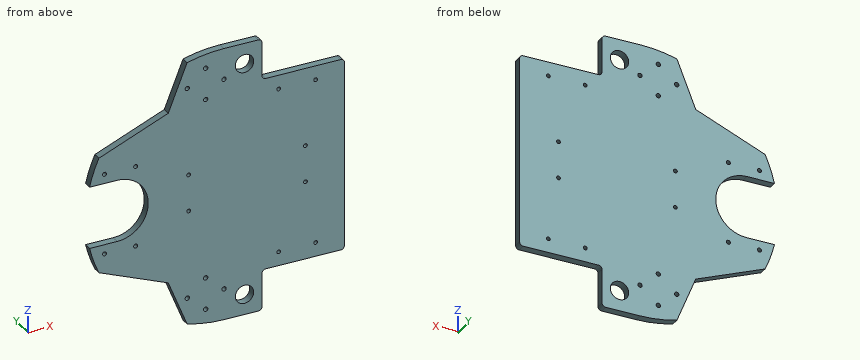
from build123d import *

# Parameters (mm, degrees)
BOSS_EXTRUDE1_DEPTH = 6.35
SKETCH8_R           = 1.651
CUT_EXTRUDE5_DEPTH  = 162.484606465
CUT_EXTRUDE6_DEPTH  = 160.416662013
SKETCH16_R          = 1.775
CUT_EXTRUDE9_DEPTH  = 160.416662013
SKETCH17_R          = 1.55
SKETCH17_R_2        = 7.5
SKETCH17_W          = 67.26995632
SKETCH17_H          = 33.5
CUT_EXTRUDE10_DEPTH = 160.416662013
FILLET1_R           = 3
SKETCH18_R          = 1.55
CUT_EXTRUDE11_DEPTH = 160.416662013


with BuildPart() as part:
    # Sketch1 → Boss-Extrude1 (new body)
    with BuildSketch(Plane(origin=(0, 0, 0), x_dir=(1, 0, 0), z_dir=(0, 1, 0))):
        with BuildLine():
            Line((-3.175, 112.5), (95.25, 112.5))
            Line((95.25, 112.5), (95.25, -112.5))
            Line((95.25, -112.5), (-3.175, -112.5))
            ThreePointArc((-3.175, -112.5), (-115.675, 0), (-3.175, 112.5))
        make_face()
    extrude(amount=-BOSS_EXTRUDE1_DEPTH)

    # Sketch8 → Cut-Extrude5 (cut, through all)
    with BuildSketch(Plane(origin=(0, 0, 0), x_dir=(1, 0, 0), z_dir=(0, 1, 0))):
        with Locations(Location((-100.5586, 33.02, 0), (0, 0, 270))):
            Circle(SKETCH8_R)
        with Locations(Location((-100.5586, -33.02, 0), (0, 0, 270))):
            Circle(SKETCH8_R)
        with Locations(Location((-75.1586, 33.02, 0), (0, 0, 270))):
            Circle(SKETCH8_R)
        with Locations(Location((-75.1586, -33.02, 0), (0, 0, 270))):
            Circle(SKETCH8_R)
        with BuildLine():
            Line((-90.2716, 25.4), (-229.776686608, 25.4))
            Line((-229.776686608, 25.4), (-229.776686608, -25.4))
            Line((-229.776686608, -25.4), (-90.2716, -25.4))
            ThreePointArc((-90.2716, -25.4), (-64.8716, 0), (-90.2716, 25.4))
        make_face()
    extrude(amount=-CUT_EXTRUDE5_DEPTH, mode=Mode.SUBTRACT)

    # Sketch9 → Cut-Extrude6 (cut, through all)
    with BuildSketch(Plane(origin=(0, 0, 0), x_dir=(1, 0, 0), z_dir=(0, 1, 0))):
        Polygon((-105.15131959, 47.508738596), (-48.53191541, 70.384462776), (-12.279886537, 160.111382848), (-19.546794421, 160.111382848), (-135.640402248, 160.111382848), (-135.640402248, 47.508738596), align=None)
        Polygon((-105.15131959, -47.508738596), (-48.53191541, -70.384462776), (-12.279886537, -160.111382848), (-135.640402248, -160.111382848), (-135.640402248, -47.508738596), align=None)
    extrude(amount=-CUT_EXTRUDE6_DEPTH, mode=Mode.SUBTRACT)

    # Sketch16 → Cut-Extrude9 (cut, through all)
    with BuildSketch(Plane(origin=(0, 0, 0), x_dir=(1, 0, 0), z_dir=(0, 1, 0))):
        with Locations(Location((-33, -87, 0), (0, 0, 270))):
            Circle(SKETCH16_R)
        with Locations(Location((-18, -100, 0), (0, 0, 270))):
            Circle(SKETCH16_R)
        with Locations(Location((-18, -74, 0), (0, 0, 270))):
            Circle(SKETCH16_R)
        with Locations(Location((-3, -87, 0), (0, 0, 270))):
            Circle(SKETCH16_R)
        with Locations(Location((-33, 87, 0), (0, 0, 270))):
            Circle(SKETCH16_R)
        with Locations(Location((-18, 100, 0), (0, 0, 270))):
            Circle(SKETCH16_R)
        with Locations(Location((-18, 74, 0), (0, 0, 270))):
            Circle(SKETCH16_R)
        with Locations(Location((-3, 87, 0), (0, 0, 270))):
            Circle(SKETCH16_R)
    extrude(amount=-CUT_EXTRUDE9_DEPTH, mode=Mode.SUBTRACT)

    # Sketch17 → Cut-Extrude10 (cut, through all)
    with BuildSketch(Plane(origin=(0, 0, 0), x_dir=(1, 0, 0), z_dir=(0, 1, 0))):
        with Locations(Location((41.62, 67.558247154, 0), (0, 0, 270))):
            Circle(SKETCH17_R)
        with Locations(Location((71.75, 67.558247154, 0), (0, 0, 270))):
            Circle(SKETCH17_R)
        with Locations(Location((41.62, -67.558247154, 0), (0, 0, 270))):
            Circle(SKETCH17_R)
        with Locations(Location((71.75, -67.558247154, 0), (0, 0, 270))):
            Circle(SKETCH17_R)
        with Locations(Location((13.687276501, 95.75, 0), (0, 0, 270))):
            Circle(SKETCH17_R_2)
        with Locations(Location((13.687276501, -95.75, 0), (0, 0, 270))):
            Circle(SKETCH17_R_2)
        with Locations((61.61502184, 95.75)):
            Rectangle(SKETCH17_W, SKETCH17_H)
        with Locations((61.61502184, -95.75)):
            Rectangle(SKETCH17_W, SKETCH17_H)
    extrude(amount=-CUT_EXTRUDE10_DEPTH, mode=Mode.SUBTRACT)

    # Fillet1
    fillet1_edges = [part.edges().sort_by_distance(p)[0] for p in [
        (95.25, -3.175, -79),
        (27.98004368, -3.175, -79),
        (27.98004368, -3.175, -112.5),
        (95.25, -3.175, 79),
        (27.98004368, -3.175, 112.5),
        (27.98004368, -3.175, 79),
    ]]
    fillet(fillet1_edges, radius=FILLET1_R)

    # Sketch18 → Cut-Extrude11 (cut, through all)
    with BuildSketch(Plane(origin=(0, 0, 0), x_dir=(1, 0, 0), z_dir=(0, 1, 0))):
        with Locations(Location((-31.919429563, 15, 0), (0, 0, 270))):
            Circle(SKETCH18_R)
        with Locations(Location((-31.919429563, -15, 0), (0, 0, 270))):
            Circle(SKETCH18_R)
        with Locations(Location((63.440570437, 15, 0), (0, 0, 270))):
            Circle(SKETCH18_R)
        with Locations(Location((63.440570437, -15, 0), (0, 0, 270))):
            Circle(SKETCH18_R)
    extrude(amount=-CUT_EXTRUDE11_DEPTH, mode=Mode.SUBTRACT)


solid = part.part
Verification items for the finished model (mm, model axes). Give positions to 0.01 mm unless a question says otherwise; leave off trailing zeros. Loops run counter-clockwise (first coordinate to the right, second up) from the corner with the lowest first, then second, coordinate; pieces in that order, holes last. Notation, with made-up numbers: (76.5, 88.25) - (86.5, 88.25) arc R15 ccw to (86.5, 95.25) - close; hole circle Ø9 at (14, 80.25). An arc over 180 degrees is marked (long way). Write item = value, one per line. Start each with the question number.
Q1. Cross-section at C-C, the plane x = -40. Enter the section's corners in (y, z).
Q2. Cross-section at D-D, the plane z = -52. Enter the section's corners in (x, y), and give its area (3 significant figures).
Q3. Thickness scan on line 1 (X direction, y = -2.5, z = 87) (3 decimals); line 2 (Z direction, x = 71.75, y = -2.5); line 3 (Z direction, x = 41, y = -3.5). Record the ranges inside material, lowest first.
Q4. Cross-section at A-A, the plane z = 95.75. Enter the section's corners in (x, y).
Q5. Cross-section at B-B, the plane y = -2.25. State how many separate pieces and enclosed holes the cut face has, and give its area (3 significant figures).
Q6. Depth check by flat-ended pin: P1, Ø1.9, axis at x = 68.5, y = -4.5, coming from the -Z side; P2, Ø1, axis at x = -23, y = -3, coming from the +Z side; P3, Ø2, axis at x = -90.5, y = -2.5, coming from the +Z side. Enter the tip coordinate at first touch or a pass-through.
Answer key:
q1.outline = (-6.35, -91.5) - (0, -91.5) - (0, 91.5) - (-6.35, 91.5) - close
q2.outline = (-94.04, -6.35) - (95.25, -6.35) - (95.25, 0) - (-94.04, 0) - close
q2.area = 1,200 mm^2
q3.line_1 = -41.819 to -34.775, -31.225 to -4.775, -1.225 to 27.98
q3.line_2 = -79 to -69.11, -66.01 to 66.01, 69.11 to 79
q3.line_3 = -79 to -68.98, -66.14 to 66.14, 68.98 to 79
q4.outline = (-38.28, -6.35) - (6.19, -6.35) - (6.19, 0) - (-38.28, 0) - close; (21.19, -6.35) - (27.98, -6.35) - (27.98, 0) - (21.19, 0) - close
q5.separate_pieces = 1
q5.enclosed_holes = 22
q5.area = 31,600 mm^2
q6.P1 = -79
q6.P2 = 110.83
q6.P3 = 53.83
